```python
from build123d import *
from build123d.topology import SkipClean

# Parameters (mm, degrees)
BOSS_EXTRUDE1_DEPTH = 41
SKETCH3_R           = 4.8
SKETCH3_R_2         = 2
BOSS_EXTRUDE2_DEPTH = 3
CUT_EXTRUDE1_START  = -8
CUT_EXTRUDE1_DEPTH  = 8
FILLET1_R           = 2


with BuildPart() as part:
    # Sketch2 → Boss-Extrude1 (new body)
    with BuildSketch(Plane.XY):
        with BuildLine():
            Line((-29.533359675, -24.776665762), (29.533359675, -24.776665762))
            ThreePointArc((29.533359675, -24.776665762), (0, -38.55), (-29.533359675, -24.776665762))
        make_face()
    extrude(amount=-BOSS_EXTRUDE1_DEPTH)

    # Sketch3 → Boss-Extrude2 (add)
    # profile 1 of 4: a face of its own
    with BuildSketch(Plane(origin=(0, -24.776665762, 0), x_dir=(1, 0, 0), z_dir=(0, 1, 0))):
        with Locations(Location((20.95, 10.5, 0), (0, 0, 270))):
            Circle(SKETCH3_R)
        with Locations(Location((20.95, 10.5, 0), (0, 0, 270))):
            Circle(SKETCH3_R_2, mode=Mode.SUBTRACT)
    # profile 2 of 4: a face of its own
    with BuildSketch(Plane(origin=(0, -24.776665762, 0), x_dir=(1, 0, 0), z_dir=(0, 1, 0))):
        with Locations(Location((20.95, 30.5, 0), (0, 0, 270))):
            Circle(SKETCH3_R)
        with Locations(Location((20.95, 30.5, 0), (0, 0, 270))):
            Circle(SKETCH3_R_2, mode=Mode.SUBTRACT)
    # profile 3 of 4: a face of its own
    with BuildSketch(Plane(origin=(0, -24.776665762, 0), x_dir=(1, 0, 0), z_dir=(0, 1, 0))):
        with Locations(Location((-20.55, 30.5, 0), (0, 0, 270))):
            Circle(SKETCH3_R)
        with Locations(Location((-20.55, 30.5, 0), (0, 0, 270))):
            Circle(SKETCH3_R_2, mode=Mode.SUBTRACT)
    # profile 4 of 4: a face of its own
    with BuildSketch(Plane(origin=(0, -24.776665762, 0), x_dir=(1, 0, 0), z_dir=(0, 1, 0))):
        with Locations(Location((-20.55, 10.5, 0), (0, 0, 270))):
            Circle(SKETCH3_R)
        with Locations(Location((-20.55, 10.5, 0), (0, 0, 270))):
            Circle(SKETCH3_R_2, mode=Mode.SUBTRACT)
    extrude(amount=BOSS_EXTRUDE2_DEPTH)

    # Sketch4 → Cut-Extrude1 (cut)
    with SkipClean():  # the faces are left unmerged after this step: merging them gives an invalid solid
        with BuildSketch(Plane(origin=(0, -24.776665762, 0), x_dir=(1, 0, 0), z_dir=(0, 1, 0)).offset(CUT_EXTRUDE1_START)):
            with BuildLine():
                Line((-18.95, 5.9745166), (-18.95, 0))
                Line((-18.95, 0), (18.95, 0))
                Line((18.95, 0), (18.95, 6.136515154))
                ThreePointArc((18.95, 6.136515154), (16.15, 10.5), (18.95, 14.863484846))
                Line((18.95, 14.863484846), (18.95, 26.136515154))
                ThreePointArc((18.95, 26.136515154), (16.15, 30.5), (18.95, 34.863484846))
                Line((18.95, 34.863484846), (18.95, 41))
                Line((18.95, 41), (-18.95, 41))
                Line((-18.95, 41), (-18.95, 35.0254834))
                ThreePointArc((-18.95, 35.0254834), (-16.630816412, 33.271281292), (-15.75, 30.5))
                ThreePointArc((-15.75, 30.5), (-16.630816412, 27.728718708), (-18.95, 25.9745166))
                Line((-18.95, 25.9745166), (-18.95, 15.0254834))
                ThreePointArc((-18.95, 15.0254834), (-16.630816412, 13.271281292), (-15.75, 10.5))
                ThreePointArc((-15.75, 10.5), (-16.630816412, 7.728718708), (-18.95, 5.9745166))
            make_face()
        extrude(amount=CUT_EXTRUDE1_DEPTH, mode=Mode.SUBTRACT)

    # Fillet1
    fillet1_edges = [part.edges().sort_by_distance(p)[0] for p in [
        (18.95, -32.776665762, -37.931742423),
        (18.95, -32.776665762, -20.5),
        (18.95, -32.776665762, -3.068257577),
        (-18.95, -32.776665762, -2.9872583),
        (-18.95, -32.776665762, -20.5),
        (-18.95, -32.776665762, -38.0127417),
    ]]
    fillet(fillet1_edges, radius=FILLET1_R)


solid = part.part
```
Geometry check sheet. Reference: the model listing, model coordinates, mm. A direction names the side the tool comes from. Give positions to 0.01 mm unless a question says otherwise; leave off trailing zeros. Order: outer loops, then holes, each group sorted by start corner. A loop starts at its lowest first (then second) coordinate and runs counter-clockwise, first axis right, second up.
1. Thickness scan on L1, parallel to X at y = -23.9, z = -30.5; L2, parallel to Y at x = -0.5, z = -29; L3, parallel to X at y = -32, z = -35. Record the ranges inside material, lowest first.
2. Release check for a two-part mould opening along Z. For faces 1 (the face through (0, -33, -41)), 2 (the face through (-18.38, -32.175, -2.797)), 3 (the face through (-22.502, -23.298, -10.934)) record: pulls with the +Z half, pulls with the -Z half, needs draft (parallel to the pull), parting line crosses it, or undercut.
3. Section check A-A, the plane y = -27.25. Enter the section's corners in (x, z).
4. Gauge pin test, flat ends, axial feed: pin 1 Ø1.5 at (x, z) = (20, -9) entering from -Y; pin 2 Ø2.5 at (x, z) = (20.95, -30.5) entering from +Y; pin 3 Ø3 at (y, z) = (-27.5, -3) entering from -X. Record the tip position at first contact, or that the pin passes through.
5. Section check D-D, the plane x = -20.55. Enter the section's corners in (y, z).
6. Access from +Z, -Z, +X, -X, +Y, -Y to the whole of each face (thin tool, end or side, straight path). Record for faces 4 (the face through (18.349, -32.206, -20.603)), 5 (the face through (18.349, -32.206, -38.003)), 6 (the face through (-18.95, -28, -3)).
7. Section check C-C, the plane x = 20.95. Enter the section's corners in (y, z).
8. Section check B-B, the plane z = -5. Enter the section's corners in (x, y).
Values follow:
1. L1: x = -25.35 to -22.55, -18.55 to -15.75, 16.15 to 18.95, 22.95 to 25.75
1. L2: y = -38.55 to -32.78
1. L3: x = -21.5 to -18.53, 18.53 to 21.5
2. face 1: pulls with the -Z half
2. face 2: needs draft
2. face 3: undercut
3. outline: (-27.27, -41) - (-18.95, -41) - (-18.95, -35.03) arc R4.8 ccw to (-18.95, -25.97) - (-18.95, -15.03) arc R4.8 ccw to (-18.95, -5.97) - (-18.95, 0) - (-27.27, 0) - close; (18.95, -41) - (27.27, -41) - (27.27, 0) - (18.95, 0) - (18.95, -6.14) arc R4.8 ccw to (18.95, -14.86) - (18.95, -26.14) arc R4.8 ccw to (18.95, -34.86) - close
4. pin 1: stops at y = -33.4
4. pin 2: stops at y = -24.78
4. pin 3: stops at x = -28.46
5. outline: (-32.62, -41) - (-24.78, -41) - (-24.78, -35.3) - (-21.78, -35.3) - (-21.78, -32.5) - (-24.78, -32.5) - (-24.78, -28.5) - (-21.78, -28.5) - (-21.78, -25.7) - (-24.78, -25.7) - (-24.78, -15.3) - (-21.78, -15.3) - (-21.78, -12.5) - (-24.78, -12.5) - (-24.78, -8.5) - (-21.78, -8.5) - (-21.78, -5.7) - (-24.78, -5.7) - (-24.78, 0) - (-32.62, 0) - close
6. face 4: +Y
6. face 5: -Z, +Y
6. face 6: +Z, +Y
7. outline: (-32.36, -41) - (-24.78, -41) - (-24.78, -35.3) - (-21.78, -35.3) - (-21.78, -32.5) - (-24.78, -32.5) - (-24.78, -28.5) - (-21.78, -28.5) - (-21.78, -25.7) - (-24.78, -25.7) - (-24.78, -15.3) - (-21.78, -15.3) - (-21.78, -12.5) - (-24.78, -12.5) - (-24.78, -8.5) - (-21.78, -8.5) - (-21.78, -5.7) - (-24.78, -5.7) - (-24.78, 0) - (-32.36, 0) - close
8. outline: (-29.53, -24.78) arc R38.55 ccw to (29.53, -24.78) - (18.95, -24.78) - (18.95, -30.78) arc R2 cw to (16.95, -32.78) - (-16.95, -32.78) arc R2 cw to (-18.95, -30.78) - (-18.95, -24.78) - close
